```python
from build123d import *

# Parameters (mm, degrees)
SKETCH_1_R          = 5
SKETCH_1_R_2        = 1.45
EXTRUDE_1_DEPTH     = 3
SKETCH_2_R          = 1.45
CUT_EXTRUDE_1_DEPTH = 74.143694192


with BuildPart() as part:
    # 草图1 → 凸台-拉伸1 (new body)
    with BuildSketch(Plane.XY):
        with BuildLine():
            Line((61.833333333, -9.830508069), (3.85, -20.644066944))
            ThreePointArc((3.85, -20.644066944), (-21, 0), (3.85, 20.644066944))
            Line((3.85, 20.644066944), (61.833333333, 9.830508069))
            ThreePointArc((61.833333333, 9.830508069), (70, 0), (61.833333333, -9.830508069))
        make_face()
        with Locations((60, 0)):
            Circle(SKETCH_1_R, mode=Mode.SUBTRACT)
        with Locations((0, 12.5)):
            Circle(SKETCH_1_R_2, mode=Mode.SUBTRACT)
        with Locations((10.825317547, 6.25)):
            Circle(SKETCH_1_R_2, mode=Mode.SUBTRACT)
        with Locations((10.825317547, -6.25)):
            Circle(SKETCH_1_R_2, mode=Mode.SUBTRACT)
        with Locations((0, -12.5)):
            Circle(SKETCH_1_R_2, mode=Mode.SUBTRACT)
        with Locations((-10.825317547, -6.25)):
            Circle(SKETCH_1_R_2, mode=Mode.SUBTRACT)
        with Locations((-10.825317547, 6.25)):
            Circle(SKETCH_1_R_2, mode=Mode.SUBTRACT)
    extrude(amount=EXTRUDE_1_DEPTH)

    # 草图2 → 切除-拉伸1 (cut, through all)
    with BuildSketch(Plane.XY.offset(3)):
        with Locations((8.75, 15.155444566)):
            Circle(SKETCH_2_R)
        with Locations((17.5, 0)):
            Circle(SKETCH_2_R)
        with Locations((8.75, -15.155444566)):
            Circle(SKETCH_2_R)
        with Locations((-8.75, -15.155444566)):
            Circle(SKETCH_2_R)
        with Locations((-17.5, 0)):
            Circle(SKETCH_2_R)
        with Locations((-8.75, 15.155444566)):
            Circle(SKETCH_2_R)
        with Locations((45, -9)):
            Circle(SKETCH_2_R)
    extrude(amount=-CUT_EXTRUDE_1_DEPTH, mode=Mode.SUBTRACT)


solid = part.part
```
Input: part model. Units: mm. Frame: model coordinates. Coordinates: 2 decimals unless noted, no trailing zeros. Write each loop counter-clockwise with the first axis right and the second up, starting at its lowest first coordinate (ties: lowest second). Pieces come first, ordered by that corner, then holes.
1) Section B-B on z = 1.8. State how many separate pieces and enclosed holes the cut face has, and give its area (3 significant figures).
2) Section A-A on y = 0. Output: boundary loops of the cut face in (x, z).
3) Mould query, pull axis X, two halves, no side actions, for faces 1 (the cylindrical face through (70, 0, 1)), 2 (the cylindrical face through (55, 0, 1)), 3 (the flat face through (15, 0, 3)), 4 (the cylindrical face through (-9.442, 6.686, 1.479)). Classes: pulls with the +X half, pulls with the -X half, needs draft (parallel to the pull), parting line crosses it, or undercut.
4) Material intervals for line 1 along Y through (x, z) = (0, 1.6); line 2 along Y through (x, z) = (-8.75, 0.9); line 3 along Y through (x, z) = (-10, 1.8), sorted ascending.
5) Pin query (flat end, axial travel): pin 1 Ø4.5 at (x, y) = (8.75, 15.16) entering from +Z. Return the tip coordinate at first contact, or that it passes through.
6) Section C-C on y = -6.25. Output: boundary loops of the cut face in (x, z).
7) Section D-D on x = 17.5. Output: boundary loops of the cut face in (y, z), and give its area (3 significant figures).
Check result:
1. separate pieces: 1
1. enclosed holes: 14
1. area: 2,580 mm2
2. outline: (-21, 0) - (-18.95, 0) - (-18.95, 3) - (-21, 3) - close; (-16.05, 0) - (16.05, 0) - (16.05, 3) - (-16.05, 3) - close; (18.95, 0) - (55, 0) - (55, 3) - (18.95, 3) - close; (65, 0) - (70, 0) - (70, 3) - (65, 3) - close
3. face 1: pulls with the +X half
3. face 2: undercut
3. face 3: needs draft
3. face 4: undercut
4. line 1: y = -21 to -13.95, -11.05 to 11.05, 13.95 to 21
4. line 2: y = -19.09 to -16.61, -13.71 to 13.71, 16.61 to 19.09
4. line 3: y = -18.47 to -15.89, -14.42 to -7.44, -5.06 to 5.06, 7.44 to 14.42, 15.89 to 18.47
5. pin 1: stops at z = 3
6. outline: (-20.05, 0) - (-12.28, 0) - (-12.28, 3) - (-20.05, 3) - close; (-9.38, 0) - (9.38, 0) - (9.38, 3) - (-9.38, 3) - close; (12.28, 0) - (67.81, 0) - (67.81, 3) - (12.28, 3) - close
7. outline: (-18.1, 0) - (-1.45, 0) - (-1.45, 3) - (-18.1, 3) - close; (1.45, 0) - (18.1, 0) - (18.1, 3) - (1.45, 3) - close
7. area: 99.9 mm2
